For this review, take the finished solid that the model builds, in its own axes (mm). A direction names the side the tool comes from. Round coordinates to 2 decimals unless told otherwise and drop trailing zeros. Loops run counter-clockwise (first coordinate to the right, second up) from the corner with the lowest first, then second, coordinate; pieces in that order, holes last. Notation, with made-up numbers: (-33, 34) -> (-11, 34) arc R28 ccw to (-11, 58) -> close; hole circle Ø2 at (58, 68). An arc over 180 degrees is marked (long way). One line per question, with ' | ' between items. Start each with the question number.
1. For faces 1 (the face through (0.3, 15.38, 10.99)), 2 (the face through (-10.901, -9, 63)), list the 3-axis set-ups (+Z, -Z, +X, -X, +Y, -Y) from which the entire face can be reached by the end or side of a thin tool; tool diameter is ignored.
2. Wall thickness on line 1 along X through (y, z) = (8.5, 18); line 2 along Y through (x, z) = (2.5, 24.5); line 3 along X through (y, z) = (15, 38): over which ranges is each line inside the solid? List them lowest first.
3. Consider section C-C (z = 114.3). Write out the cut boundary in (x, y), and give its area (3 significant figures).
4. Consider section B-B (x = -6). Write out the cut boundary in (y, z).
5. Draft analysis for pull direction Z (two halves, no side actions). For faces 3 (the face through (-12, -9, 127)), 4 (the face through (11.959, -10, 63)), 5 (the face through (0.3, -34.15, 10.99)), 6 (the face through (0.3, -34.15, 36.39)), state which applies: pulls with the +Z half, pulls with the -Z half, needs draft (parallel to the pull), parting line crosses it, or undercut.
6. Consider section D-D (z = 20.5). Write out the cut boundary in (x, y).
7. Consider section A-A (y = -25). Write out the cut boundary in (x, z), and give its area (3 significant figures).
Autodesk Inventor part; units mm, degrees
ref_plane "YZ Plane" through (0, 0, 0) normal (1, 0, 0) x (0, 1, 0)
ref_plane "XZ Plane" through (0, 0, 0) normal (0, 1, 0) x (-1, 0, 0)
ref_plane "XY Plane" through (0, 0, 0) normal (0, 0, 1) x (1, 0, 0)
sketch "Sketch1" plane through (0, 0, 0) normal (0, 0, 1) x (1, 0, 0)
  line L0 (-12.1708, 16.0073) -> (13.2292, 16.0073)
  line L1 (13.2292, 16.0073) -> (13.2292, -34.7927)
  line L2 (13.2292, -34.7927) -> (-12.1708, -34.7927)
  line L3 (-12.1708, -34.7927) -> (-12.1708, 16.0073)
  line L4 (11.9592, 14.7373) -> (-10.9008, 14.7373)
  line L5 (-10.9008, 14.7373) -> (-10.9008, -33.5227)
  line L6 (-10.9008, -33.5227) -> (11.9592, -33.5227)
  line L7 (11.9592, -33.5227) -> (11.9592, 14.7373)
  point P0 (0, 0)
  dimension "d0" = 25.4
  dimension "d1" = 50.8
  dimension "d2" = 1.27
extrude "Extrusion1" add sketch "Sketch1" along normal blind 127
sketch "Sketch2" plane through (-12.1708, 16.0073, 0) normal (0, 1, 0) x (1, 0, 0)
  circle A0 centre (12.7, -12.7) radius 1.7272
  line L0 (25.4, 0) -> (0, 0)
  line L1 (0, 0) -> (0, -127)
  point P0 (12.1708, 0)
  dimension "d5" = 3.4544
  dimension "d6" = 12.7
  dimension "d7" = 12.7
extrude "Extrusion2" cut sketch "Sketch2" against normal through all
pattern_linear "Rectangular Pattern1" count 13 spacing 25.4 along (0, 0, 1) of "Extrusion2"
equation "\"d3\" = d13"
equation "\"d10\" = d14"
equation "\"d13\" = 127"
equation "\"d14\" = d13"
properties part number "VerseFrame 5in STOCK"
Answer block:
1) face 1: +Y, -Y | face 2: +Z, -Z
2) line 1: x = -12.17 to -10.9, 11.96 to 13.23 | line 2: y = -34.79 to -33.52, 14.74 to 16.01 | line 3: x = -12.17 to -1.2, 2.25 to 13.23
3) outline: (-12.17, -34.79) -> (-1.2, -34.79) -> (-1.2, -33.52) -> (-10.9, -33.52) -> (-10.9, 14.74) -> (-1.2, 14.74) -> (-1.2, 16.01) -> (-12.17, 16.01) -> close; (2.26, -34.79) -> (13.23, -34.79) -> (13.23, 16.01) -> (2.26, 16.01) -> (2.26, 14.74) -> (11.96, 14.74) -> (11.96, -33.52) -> (2.26, -33.52) -> close | area: 178 mm2
4) outline: (-34.79, 0) -> (-33.52, 0) -> (-33.52, 127) -> (-34.79, 127) -> close; (14.74, 0) -> (16.01, 0) -> (16.01, 127) -> (14.74, 127) -> close
5) face 3: pulls with the +Z half | face 4: needs draft | face 5: undercut | face 6: undercut
6) outline: (-12.17, -34.79) -> (13.23, -34.79) -> (13.23, 16.01) -> (-12.17, 16.01) -> close; hole (-10.9, -33.52) -> (11.96, -33.52) -> (11.96, 14.74) -> (-10.9, 14.74) -> close
7) outline: (-12.17, 0) -> (-10.9, 0) -> (-10.9, 127) -> (-12.17, 127) -> close; (11.96, 0) -> (13.23, 0) -> (13.23, 127) -> (11.96, 127) -> close | area: 323 mm2
